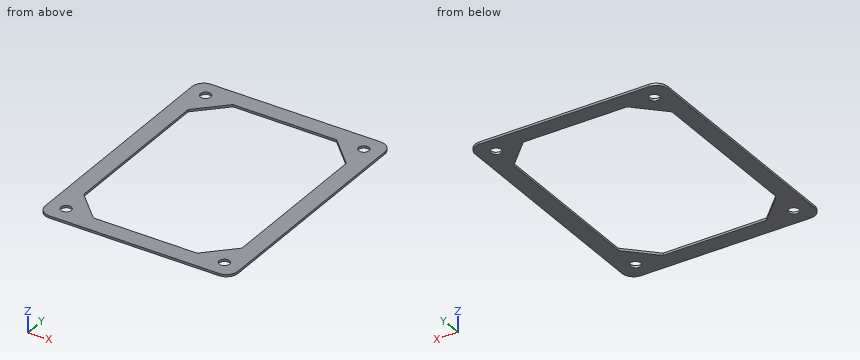
from build123d import *

# Parameters (mm, degrees)
SKETCH1_R           = 2.286
BOSS_EXTRUDE1_DEPTH = 1


with BuildPart() as part:
    # Sketch1 → Boss-Extrude1 (new body)
    with BuildSketch(Plane.XY):
        with BuildLine():
            Line((1.27, -104.14), (1.27, -3.81))
            ThreePointArc((1.27, -3.81), (-0.217897552, -0.217897552), (-3.81, 1.27))
            Line((-3.81, 1.27), (-78.74, 1.27))
            ThreePointArc((-78.74, 1.27), (-82.332102448, -0.217897552), (-83.82, -3.81))
            Line((-83.82, -3.81), (-83.82, -104.14))
            ThreePointArc((-83.82, -104.14), (-82.332102448, -107.732102448), (-78.74, -109.22))
            Line((-78.74, -109.22), (-3.81, -109.22))
            ThreePointArc((-3.81, -109.22), (-0.217897552, -107.732102448), (1.27, -104.14))
        make_face()
        with Locations((-76.2, -6.35)):
            Circle(SKETCH1_R, mode=Mode.SUBTRACT)
        with Locations((-76.2, -101.6)):
            Circle(SKETCH1_R, mode=Mode.SUBTRACT)
        with Locations((-6.35, -101.6)):
            Circle(SKETCH1_R, mode=Mode.SUBTRACT)
        with Locations((-6.35, -6.35)):
            Circle(SKETCH1_R, mode=Mode.SUBTRACT)
        Polygon((-76.2, -18.35), (-64.2, -6.35), (-18.35, -6.35), (-6.35, -18.35), (-6.35, -89.6), (-18.35, -101.6), (-64.2, -101.6), (-76.2, -89.6), align=None, mode=Mode.SUBTRACT)
    extrude(amount=BOSS_EXTRUDE1_DEPTH)


solid = part.part
Model file for the job. Use its own axes, mm. Round coordinates to 2 decimals unless told otherwise and drop trailing zeros. Order: outer loops, then holes, each group sorted by start corner. A loop starts at its lowest first (then second) coordinate and runs counter-clockwise, first axis right, second up.
(1) Pin check, flat tip, straight feed: pin 1 (10 mm diameter, centred on x = -70, y = -17, fed in from +Z). Stop position of the tip, or through.
(2) Band-saw the part on B-B (y = -68). List the corners of the cut face in (x, z).
(3) Drill centre lines: line 1 (Y direction, x = -47, z = 0.9); line 2 (X direction, y = -59.5, z = 0.2); line 3 (Y direction, x = -69, z = 0.9). Where is each one in solid material? Low to high.
(4) Band-saw the part on C-C (z = 0.65). List the corners of the cut face in (x, y), then the cut area to 3 significant figures.
(5) Band-saw the part on A-A (x = -42.5). List the corners of the cut face in (y, z).
Verdict:
1. pin 1: stops at z = 1
2. outline: (-83.82, 0) - (-76.2, 0) - (-76.2, 1) - (-83.82, 1) - close; (-6.35, 0) - (1.27, 0) - (1.27, 1) - (-6.35, 1) - close
3. line 1: y = -109.22 to -101.6, -6.35 to 1.27
3. line 2: x = -83.82 to -76.2, -6.35 to 1.27
3. line 3: y = -109.22 to -96.8, -11.15 to 1.27
4. outline: (-83.82, -104.14) arc R5.08 ccw to (-78.74, -109.22) - (-3.81, -109.22) arc R5.08 ccw to (1.27, -104.14) - (1.27, -3.81) arc R5.08 ccw to (-3.81, 1.27) - (-78.74, 1.27) arc R5.08 ccw to (-83.82, -3.81) - close; hole circle Ø4.57 at (-76.2, -101.6); hole circle Ø4.57 at (-76.2, -6.35); hole (-76.2, -89.6) - (-64.2, -101.6) - (-18.35, -101.6) - (-6.35, -89.6) - (-6.35, -18.35) - (-18.35, -6.35) - (-64.2, -6.35) - (-76.2, -18.35) - close; hole circle Ø4.57 at (-6.35, -101.6); hole circle Ø4.57 at (-6.35, -6.35)
4. area: 2,950 mm2
5. outline: (-109.22, 0) - (-101.6, 0) - (-101.6, 1) - (-109.22, 1) - close; (-6.35, 0) - (1.27, 0) - (1.27, 1) - (-6.35, 1) - close
